Design review of the part built by this model. Coordinates are the model's own, in mm. A direction names the side the tool comes from. Give positions to 0.01 mm unless a question says otherwise; leave off trailing zeros. Loops run counter-clockwise (first coordinate to the right, second up) from the corner with the lowest first, then second, coordinate; pieces in that order, holes last. Notation, with made-up numbers: M 17,7.5 L 76,7.5 A21 cw 76,24.5 Z; hole C -5.75,-12.5 d2. An arc over 180 degrees is marked long. Answer as CSV lines item,"result".
```python
from build123d import *

# Parameters (mm, degrees)
CUT_EXTRUDE1_DEPTH = 1.34
CHAMFER1_SIZE      = 0.25
FILLET1_R          = 0.5
FILLET2_R          = 0.5


with BuildPart() as part:
    # Sketch1 → Revolve1 (revolve)
    with BuildSketch(Plane.XY):
        with BuildLine():
            Line((0, -4), (1.5, -4))
            Line((1.5, -4), (1.5, 0))
            Line((1.5, 0), (3.45, 0))
            Line((3.45, 0), (3.45, 0.475))
            ThreePointArc((3.45, 0.475), (1.866355071, 1.529728066), (0, 1.9))
            Line((0, 1.9), (0, -4))
        make_face()
    revolve(axis=Axis((0, -2.988815789, 0), (0, 1, 0)))

    # Sketch3 → Cut-Extrude1 (cut)
    with BuildSketch(Plane(origin=(0, 1.9, 0), x_dir=(-1, 0, 0), z_dir=(0, 1, 0))):
        Polygon((-0.3625, 1.45), (0.3625, 1.45), (0.3625, 0.3625), (1.45, 0.3625), (1.45, -0.3625), (0.3625, -0.3625), (0.3625, -1.45), (-0.3625, -1.45), (-0.3625, -0.3625), (-1.45, -0.3625), (-1.45, 0.3625), (-0.3625, 0.3625), align=None)
    extrude(amount=-CUT_EXTRUDE1_DEPTH, mode=Mode.SUBTRACT)

    # Chamfer1
    chamfer1_edges = [part.edges().sort_by_distance(p)[0] for p in [
        (-1.5, -4, 0),
    ]]
    chamfer(chamfer1_edges, length=CHAMFER1_SIZE)

    # Fillet1
    fillet1_edges = [part.edges().sort_by_distance(p)[0] for p in [
        (-3.45, 0.475, 0),
    ]]
    fillet(fillet1_edges, radius=FILLET1_R)

    # Fillet2
    fillet2_edges = [part.edges().sort_by_distance(p)[0] for p in [
        (0.3625, 1.216523373, 0.3625),
        (-0.3625, 1.216523373, 0.3625),
        (-0.3625, 1.216523373, -0.3625),
        (0.3625, 1.216523373, -0.3625),
    ]]
    fillet(fillet2_edges, radius=FILLET2_R)


solid = part.part
```
1. For P1, Ø0.5, axis at x = 1, y = 1.5, coming from the -Z side; P2, Ø0.8, axis at x = 0, y = 1, coming from the +Z side; P3, Ø0.6, axis at x = -1, y = 1.5, coming from the +Z side, all flat-tipped, find the tip position at first contact; note any pin that passes through.
Answer block:
P1,"z = -2.23"
P2,"z = 3.32"
P3,"z = 2.33"
2. For faces 1 (the flat face through (-1.5, 0, 0.7)), 2 (the flat face through (0, 0.56, 0)), 3 (the flat face through (0, -4, 0)), list the 3-axis set-ups (+Z, -Z, +X, -X, +Y, -Y) from which the entire face can be reached by the end or side of a thin tool; tool diameter is ignored.
Answer block:
face 1,"-Y"
face 2,"+Y"
face 3,"+Z, -Z, +X, -X, -Y"
3. We need section B-B, the plane y = -3.05. Write out the cut boundary in (x, z), plus the area to 3 significant figures.
Answer block:
outline,"C 0,0 d3"
area,"7.07 mm²"
4. We need section A-A, the plane y = 0.9. Write out the cut boundary in (x, z).
Answer block:
outline,"C 0,0 d5.93; hole M -1.45,-0.36 L -0.86,-0.36 A0.5 cw -0.36,-0.86 L -0.36,-1.45 L 0.36,-1.45 L 0.36,-0.86 A0.5 cw 0.86,-0.36 L 1.45,-0.36 L 1.45,0.36 L 0.86,0.36 A0.5 cw 0.36,0.86 L 0.36,1.45 L -0.36,1.45 L -0.36,0.86 A0.5 cw -0.86,0.36 L -1.45,0.36 Z"
5. To check wall thickness, follow L1, parallel to X at y = 0.8, z = -1; L2, parallel to Y at x = 0.5, z = 0; L3, parallel to Y at x = 1.25, z = -1.75. State the ranges of each line that lie inside material, in increasing order. Write a range as [from, to].
Answer block:
L1,"[-2.92, -0.36], [0.36, 2.92]"
L2,"[-4, 0.56]"
L3,"[0, 1.4]"
